Design review of the part built by this model. Coordinates are the model's own, in mm. Give positions to 0.01 mm unless a question says otherwise; leave off trailing zeros. Write each loop counter-clockwise with the first axis right and the second up, starting at its lowest first coordinate (ties: lowest second). Pieces come first, ordered by that corner, then holes. Notation, with made-up numbers: (-30, 42.5) -> (-11, 42.5) arc R15 cw to (-11, 64.5) -> close; hole circle Ø11 at (29.25, 79.5). An arc over 180 degrees is marked (long way). Write each question's results on one line, items separated by ' | '. Start each with the question number.
(1) Mouldability with a two-part tool opening along Y and no side actions: class faces 1 (the face through (0, 0, 0)), 2 (the face through (22.295, -24.444, 0.246)), 3 (the face through (20.65, 22.48, 0.25)), 4 (the face through (24.05, -30.47, 0.64)) as released by +Y, released by -Y, zero draft, split by the parting line, or undercut.
(2) To check wall thickness, follow probe 1 along Y at (x, z) = (19.1, 0.25); probe 2 along X at (y, z) = (-28, 0.75); probe 3 along X at (y, z) = (27, 0.95). State the ranges of each line that lie inside material, in increasing order.
(3) Take a section at C-C (z = 1). State the section outline as (x, y) points.
(4) Clearance check with flat-ended pins moving along their axes: pin 1 (7.5 mm diameter, centred on x = -19.1, y = 25.45, fed in from +Z); pin 2 (7.5 mm diameter, centred on x = 19.1, y = 25.45, fed in from -Z); pin 3 (4 mm diameter, centred on x = -19.1, y = -25.45, fed in from +Z). State where each tip first meets the part, or that it passes through.
(5) Take a section at A-A (x = 19.1). State the section outline as (y, z) points.
(6) Take a section at B-B (y = 25.45). State the section outline as (x, z) points, plus the area to 3 significant figures.
from build123d import *

# Parameters (mm, degrees)
F0_R     = 3.35
F1_DEPTH = 1.5
F2_SIZE  = 1
F3_SIZE  = 0.2


with BuildPart() as f1:
    # F0 (on Top) → F1 (new body)
    with BuildSketch(Plane.XY):
        with BuildLine():
            Line((20.55, 31.9), (-20.55, 31.9))
            ThreePointArc((-20.55, 31.9), (-24.085534, 30.435534), (-25.55, 26.9))
            Line((-25.55, 26.9), (-25.55, -26.9))
            ThreePointArc((-25.55, -26.9), (-24.085534, -30.435534), (-20.55, -31.9))
            Line((-20.55, -31.9), (20.55, -31.9))
            ThreePointArc((20.55, -31.9), (24.085534, -30.435534), (25.55, -26.9))
            Line((25.55, -26.9), (25.55, 26.9))
            ThreePointArc((25.55, 26.9), (24.085534, 30.435534), (20.55, 31.9))
        make_face()
        with Locations((-19.1, -25.45)):
            Circle(F0_R, mode=Mode.SUBTRACT)
        with Locations((19.1, -25.45)):
            Circle(F0_R, mode=Mode.SUBTRACT)
        with Locations((-19.1, 25.45)):
            Circle(F0_R, mode=Mode.SUBTRACT)
        with Locations((19.1, 25.45)):
            Circle(F0_R, mode=Mode.SUBTRACT)
    extrude(amount=F1_DEPTH)

    # F2
    f2_edges = [f1.edges().sort_by_distance(p)[0] for p in [
        (-22.45, 25.45, 1.5),
        (15.75, 25.45, 1.5),
        (15.75, -25.45, 1.5),
        (-22.45, -25.45, 1.5),
    ]]
    chamfer(f2_edges, length=F2_SIZE)

    # F3
    f3_edges = [f1.edges().sort_by_distance(p)[0] for p in [
        (-24.085534, 30.435534, 1.5),
        (-25.55, 0, 1.5),
        (-24.085534, -30.435534, 1.5),
        (0, 31.9, 1.5),
        (24.085534, 30.435534, 1.5),
        (25.55, 0, 1.5),
        (24.085534, -30.435534, 1.5),
        (0, -31.9, 1.5),
    ]]
    chamfer(f3_edges, length=F3_SIZE)


solid = f1.part
Report:
1) face 1: zero draft | face 2: undercut | face 3: undercut | face 4: released by -Y
2) probe 1: -31.9 to -28.8, -22.1 to 22.1, 28.8 to 31.9 | probe 2: -25.43 to -21.64, -16.56 to 16.56, 21.64 to 25.43 | probe 3: -25.55 to -22.57, -15.63 to 15.63, 22.57 to 25.55
3) outline: (-25.55, -26.9) arc R5 ccw to (-20.55, -31.9) -> (20.55, -31.9) arc R5 ccw to (25.55, -26.9) -> (25.55, 26.9) arc R5 ccw to (20.55, 31.9) -> (-20.55, 31.9) arc R5 ccw to (-25.55, 26.9) -> close; hole circle Ø7.7 at (-19.1, -25.45); hole circle Ø7.7 at (-19.1, 25.45); hole circle Ø7.7 at (19.1, -25.45); hole circle Ø7.7 at (19.1, 25.45)
4) pin 1: z = 0.9 | pin 2: z = 0 | pin 3: through
5) outline: (-31.9, 0) -> (-28.8, 0) -> (-28.8, 0.5) -> (-29.8, 1.5) -> (-31.7, 1.5) -> (-31.9, 1.3) -> close; (-22.1, 0) -> (22.1, 0) -> (22.1, 0.5) -> (21.1, 1.5) -> (-21.1, 1.5) -> (-22.1, 0.5) -> close; (28.8, 0) -> (31.9, 0) -> (31.9, 1.3) -> (31.7, 1.5) -> (29.8, 1.5) -> (28.8, 0.5) -> close
6) outline: (-25.55, 0) -> (-22.45, 0) -> (-22.45, 0.5) -> (-23.45, 1.5) -> (-25.35, 1.5) -> (-25.55, 1.3) -> close; (-15.75, 0) -> (15.75, 0) -> (15.75, 0.5) -> (14.75, 1.5) -> (-14.75, 1.5) -> (-15.75, 0.5) -> close; (22.45, 0) -> (25.55, 0) -> (25.55, 1.3) -> (25.35, 1.5) -> (23.45, 1.5) -> (22.45, 0.5) -> close | area: 54.5 mm2
